```python
from build123d import *

# Parameters (mm, degrees)
BOSS_EXTRUDE1_DEPTH = 100
SKETCH2_W           = 10
SKETCH2_H           = 450
BOSS_EXTRUDE2_DEPTH = 20
SKETCH3_R           = 2
CUT_EXTRUDE1_DEPTH  = 483.494777174


with BuildPart() as part:
    # Sketch1 → Boss-Extrude1 (new body)
    with BuildSketch(Plane(origin=(0, 0, 0), x_dir=(1, 0, 0), z_dir=(0, 1, 0))):
        Polygon((100, -41.421356237), (100, 41.421356237), (41.421356237, 100), (-41.421356237, 100), (-100, 41.421356237), (-100, -41.421356237), (-41.421356237, -100), (41.421356237, -100), align=None)
    extrude(amount=BOSS_EXTRUDE1_DEPTH)

    # Sketch2 → Boss-Extrude2 (add)
    with BuildSketch(Plane(origin=(0, 100, 0), x_dir=(1, 0, 0), z_dir=(0, 1, 0))):
        with Locations((-21.1, -225)):
            Rectangle(SKETCH2_W, SKETCH2_H)
        with Locations((21.1, -225)):
            Rectangle(SKETCH2_W, SKETCH2_H)
    extrude(amount=BOSS_EXTRUDE2_DEPTH)

    # Sketch3 → Cut-Extrude1 (cut, through all)
    with BuildSketch(Plane.ZY.offset(26.1)):
        with Locations((438, 110)):
            Circle(SKETCH3_R)
        with Locations((420, 110)):
            Circle(SKETCH3_R)
        with Locations((402, 110)):
            Circle(SKETCH3_R)
    extrude(amount=-CUT_EXTRUDE1_DEPTH, mode=Mode.SUBTRACT)


solid = part.part
```
The listing builds one solid part. Answer for the finished solid, in the listing's coordinates (mm). A direction names the side the tool comes from. Give positions to 0.01 mm unless a question says otherwise; leave off trailing zeros. Order: outer loops, then holes, each group sorted by start corner. A loop starts at its lowest first (then second) coordinate and runs counter-clockwise, first axis right, second up. Notation, with made-up numbers: (84.5, -25) -> (140.5, -25) arc R26 cw to (140.5, 12) -> close; hole circle Ø1 at (5.25, 16.5). An arc over 180 degrees is marked (long way). One line per item, written item: value.
1) Find section D-D, the plane x = -74. Determine the outline of the cut face in (y, z), plus the area to 3 significant figures.
Reported:
outline: (0, -67.42) -> (100, -67.42) -> (100, 67.42) -> (0, 67.42) -> close
area: 13,500 mm^2
2) Find section A-A, the plane z = 321. Determine the outline of the cut face in (x, y), plus the area to 3 significant figures.
Reported:
outline: (-26.1, 100) -> (-16.1, 100) -> (-16.1, 120) -> (-26.1, 120) -> close; (16.1, 100) -> (26.1, 100) -> (26.1, 120) -> (16.1, 120) -> close
area: 400 mm^2
3) Find section B-B, the plane y = 50.5. Determine the outline of the cut face in (x, z).
Reported:
outline: (-100, -41.42) -> (-41.42, -100) -> (41.42, -100) -> (100, -41.42) -> (100, 41.42) -> (41.42, 100) -> (-41.42, 100) -> (-100, 41.42) -> close
4) Find the intervals of material crossed by line 1 (Y direction, x = -23.5, z = 420); line 2 (X direction, y = 109.5, z = 383); line 3 (Z direction, x = -24.5, y = 25.5), in increasing order.
Reported:
line 1: y = 100 to 108, 112 to 120
line 2: x = -26.1 to -16.1, 16.1 to 26.1
line 3: z = -100 to 100
5) A tool of negligible diameter and unlimited length cuts with its end or side. For faces 1 (the flat face through (-1, 49, 100)), 2 (the flat face through (-70.3, 49.3, -71.12)), 3 (the flat face through (16.1, 110, 228)), 4 (the flat face through (21, 110, 0)), from which of +Z, -Z, +X, -X, +Y, -Y can it reach the whole face along a straight path? Write none if from no direction.
Reported:
face 1: +Z, +X, -X, -Y
face 2: -Z, -X, +Y, -Y
face 3: +Z, -Z, +Y
face 4: -Z, +X, -X, +Y
6) Flat-ended cylindrical pins translate along their axes: P1, Ø8, axis at x = 23, z = 188, coming from the -Y side; P2, Ø6, axis at y = 108, z = 287, coming from the +X side; P3, Ø8, axis at x = 23, y = 113.5, coming from the -Z side. Find the tip coordinate at first contact, or state that the pin passes through.
Reported:
P1: stops at y = 100
P2: stops at x = 26.1
P3: stops at z = 0
7) Find section C-C, the plane z = 6.5. Determine the outline of the cut face in (x, y).
Reported:
outline: (-100, 0) -> (100, 0) -> (100, 100) -> (26.1, 100) -> (26.1, 120) -> (16.1, 120) -> (16.1, 100) -> (-16.1, 100) -> (-16.1, 120) -> (-26.1, 120) -> (-26.1, 100) -> (-100, 100) -> close
8) Determine the mould class of faces 5 (the flat face through (26.1, 110, 228)), 6 (the flat face through (1, 49, -100)), 7 (the flat face through (-16.1, 110, 228)) for opening direction X: pulls with the +X half, pulls with the -X half, needs draft (parallel to the pull), parting line crosses it, or undercut.
Reported:
face 5: pulls with the +X half
face 6: needs draft
face 7: undercut
